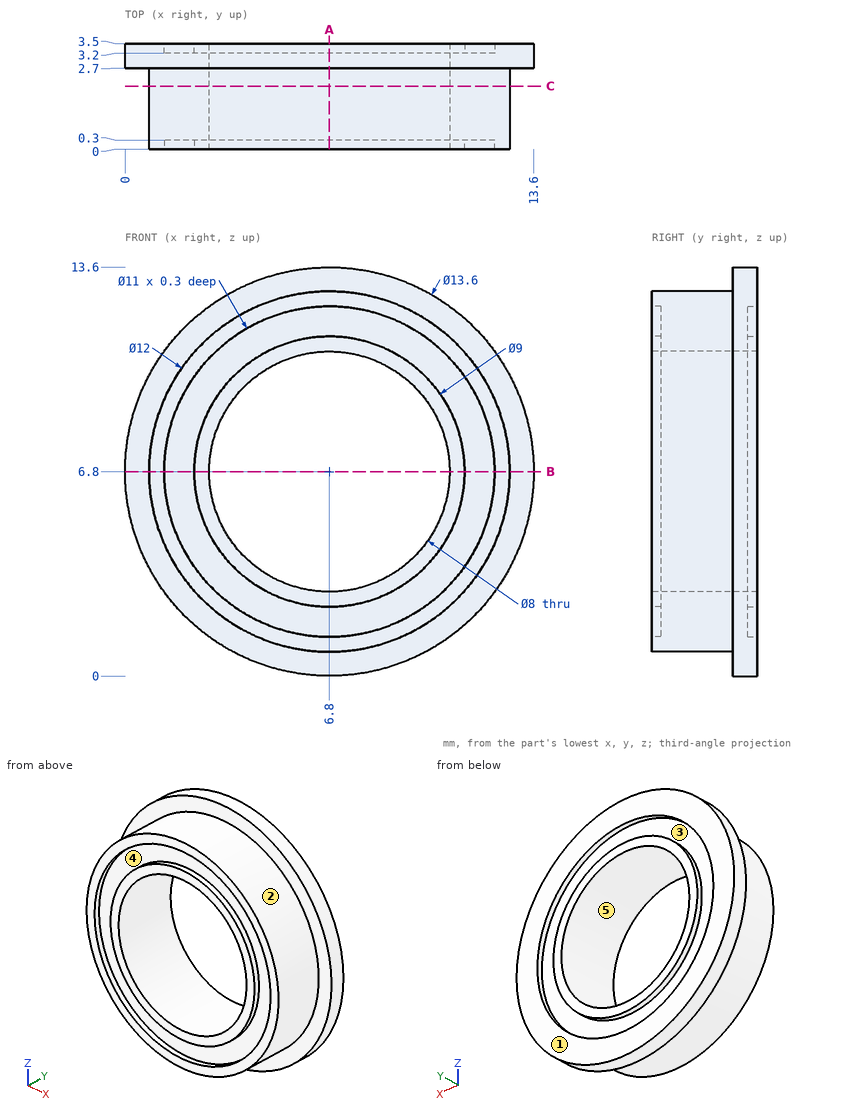
Answer from the drawing. Dimensions are ordinates in mm from the lowest x, y and z of the part. A direction names the side the tool comes from. Coordinates: 2 decimals unless noted, no trailing zeros. Write each loop counter-clockwise with the first axis right and the second up, starting at its lowest first coordinate (ties: lowest second). Pieces come first, ordered by that corner, then holes. Notation, with made-up numbers: (55.25, 83.25) - (66.25, 83.25) arc R18 ccw to (66.25, 89.25) - close; hole circle Ø8 at (-34.5, -30.75). An arc over 180 degrees is marked (long way). Return JSON: item names as keys, results as strings. Group by question number.
Q1. The part is cut by section B-B on z = 6.8. Write down the section's boundary in (x, y).
Q2. The part is cut by section C-C on y = 2.1. Write down the section's boundary in (x, z), and give its area (3 significant figures).
Q3. For a pull along X with two mould halves and no side action, classify the marked faces 1, 2 and 3 as +X half, -X half, draft (parallel to the pull), parting line (faces both ways), or undercut.
Q4. Which of the six approach directions +Z, -Z, +X, -X, +Y, -Y give full straight-line access (tool end or side, diameter ignored) to the marked faces 4 and 5?
Q5. The part is cut by section A-A on x = 6.8. Write down the section's boundary in (y, z), and give its area (3 significant figures).
Q6. Find the intervals of material crossed by line 1 along Z through (x, y) = (6.8, 0.15); line 2 along Z through (x, y) = (6.8, 3.45); line 3 along Z through (x, y) = (6.8, 1.45), in increasing order. Write a range as [from, to].
Q7. A flat-ended cylindrical pin translates along its axis: pin 1 Ø1.5 at (y, z) = (2.5, 8) entering from +X. Find the tip coordinate at first contact, or state that the pin passes through.
Evaluation:
{
 "1": {"outline": "(0, 2.7) - (0.8, 2.7) - (0.8, 0) - (1.3, 0) - (1.3, 0.3) - (2.3, 0.3) - (2.3, 0) - (2.8, 0) - (2.8, 3.5) - (2.3, 3.5) - (2.3, 3.2) - (1.3, 3.2) - (1.3, 3.5) - (0, 3.5) - close; (10.8, 0) - (11.3, 0) - (11.3, 0.3) - (12.3, 0.3) - (12.3, 0) - (12.8, 0) - (12.8, 2.7) - (13.6, 2.7) - (13.6, 3.5) - (12.3, 3.5) - (12.3, 3.2) - (11.3, 3.2) - (11.3, 3.5) - (10.8, 3.5) - close"},
 "2": {"outline": "circle Ø12 at (6.8, 6.8); hole circle Ø8 at (6.8, 6.8)", "area": "62.8 mm2"},
 "3": {"face 1": "draft", "face 2": "parting line", "face 3": "undercut"},
 "4": {"face 4": "-Y", "face 5": "+Y, -Y"},
 "5": {"outline": "(0, 0.8) - (2.7, 0.8) - (2.7, 0) - (3.5, 0) - (3.5, 1.3) - (3.2, 1.3) - (3.2, 2.3) - (3.5, 2.3) - (3.5, 2.8) - (0, 2.8) - (0, 2.3) - (0.3, 2.3) - (0.3, 1.3) - (0, 1.3) - close; (0, 10.8) - (3.5, 10.8) - (3.5, 11.3) - (3.2, 11.3) - (3.2, 12.3) - (3.5, 12.3) - (3.5, 13.6) - (2.7, 13.6) - (2.7, 12.8) - (0, 12.8) - (0, 12.3) - (0.3, 12.3) - (0.3, 11.3) - (0, 11.3) - close", "area": "14.1 mm2"},
 "6": {"line 1": "z = [0.8, 1.3], [2.3, 2.8], [10.8, 11.3], [12.3, 12.8]", "line 2": "z = [0, 1.3], [2.3, 2.8], [10.8, 11.3], [12.3, 13.6]", "line 3": "z = [0.8, 2.8], [10.8, 12.8]"},
 "7": {"pin 1": "stops at x = 13.58"}
}
